Can you work these out from the model? Positions are in its coordinate system, mm. A direction names the side the tool comes from. Give positions to 0.01 mm unless a question says otherwise; leave off trailing zeros. Order: outer loops, then holes, each group sorted by start corner. A loop starts at its lowest first (then second) coordinate and runs counter-clockwise, first axis right, second up. Notation, with made-up numbers: (50, -3) - (76, -3) arc R32 cw to (76, 30) - close; hole circle Ø3 at (58, 86.5). An arc over 180 degrees is marked (long way). Answer as CSV lines item,"result".
```python
from build123d import *

# Parameters (mm, degrees)
SKETCH1_W                      = 55
SKETCH1_H                      = 39.55
SKETCH1_R                      = 7.5
BOSS_EXTRUDE1_DEPTH            = 45
SKETCH3_R                      = 4
CUT_EXTRUDE1_DEPTH             = 9.55
SKETCH4_W                      = 11
SKETCH4_H                      = 20
CUT_EXTRUDE2_DEPTH             = 65.21216785
M3_CLEARANCE_HOLE1_D           = 3.4
M3_CLEARANCE_HOLE1_DEPTH       = 32
M3_CLEARANCE_HOLE1_CSINK_D     = 3.45
M3_CLEARANCE_HOLE1_CSINK_ANGLE = 90
M3_CLEARANCE_HOLE1_TIP         = 1.021463052
SKETCH8_W                      = 9
SKETCH8_H                      = 4.627198444
CUT_EXTRUDE3_DEPTH             = 65.21216785
FILLET1_R                      = 10
FILLET2_R                      = 2
FILLET3_R                      = 6
FILLET4_R                      = 13


with BuildPart() as part:
    # Sketch1 → Boss-Extrude1 (new body)
    with BuildSketch(Plane.XY):
        with Locations((-7.5, 9.775)):
            Rectangle(SKETCH1_W, SKETCH1_H)
        with Locations((7.34, 19.55)):
            Circle(SKETCH1_R, mode=Mode.SUBTRACT)
    extrude(amount=-BOSS_EXTRUDE1_DEPTH)

    # Sketch3 → Cut-Extrude1 (cut)
    with BuildSketch(Plane.XZ.offset(10)):
        with Locations((7.34, -11.25)):
            Circle(SKETCH3_R)
        with Locations((7.34, -33.75)):
            Circle(SKETCH3_R)
    extrude(amount=-CUT_EXTRUDE1_DEPTH, mode=Mode.SUBTRACT)

    # Sketch4 → Cut-Extrude2 (cut, through all)
    with BuildSketch(Plane.XY):
        with Locations((-26.5, 0)):
            Rectangle(SKETCH4_W, SKETCH4_H)
    extrude(amount=-CUT_EXTRUDE2_DEPTH, mode=Mode.SUBTRACT)

    # M3 Clearance Hole1
    with Locations(Plane(origin=(-35, -1, -36), x_dir=(0, 0, -1), z_dir=(-1, 0, 0))):
        with Locations((0, 0), (-27, 0)):
            CounterSinkHole(M3_CLEARANCE_HOLE1_D / 2, M3_CLEARANCE_HOLE1_CSINK_D / 2, depth=M3_CLEARANCE_HOLE1_DEPTH, counter_sink_angle=M3_CLEARANCE_HOLE1_CSINK_ANGLE)
            with Locations((0, 0, -(M3_CLEARANCE_HOLE1_DEPTH + M3_CLEARANCE_HOLE1_TIP / 2))):  # 118° drill point
                Cone(0, M3_CLEARANCE_HOLE1_D / 2, M3_CLEARANCE_HOLE1_TIP, mode=Mode.SUBTRACT)

    # Sketch8 → Cut-Extrude3 (cut, through all)
    with BuildSketch(Plane.XY):
        with Locations((-26.66, 24.492052806)):
            Rectangle(SKETCH8_W, SKETCH8_H)
    extrude(amount=-CUT_EXTRUDE3_DEPTH, mode=Mode.SUBTRACT)

    # Fillet1
    # the kernel refuses this fillet: 10 mm, written as the material it takes off along each edge
    with BuildSketch(Plane(origin=(-46, -10, 0), x_dir=(0, 1, 0), z_dir=(1, 0, 0))) as fillet1_piece_1:
        with BuildLine():
            CenterArc((FILLET1_R, -FILLET1_R), FILLET1_R, 90, 90)
            Line((0, -FILLET1_R), (0, 0))
            Line((0, 0), (FILLET1_R, 0))
        make_face()
    extrude(amount=91, mode=Mode.SUBTRACT)
    with BuildSketch(Plane(origin=(-46, -10, -45), x_dir=(0, 1, 0), z_dir=(1, 0, 0))) as fillet1_piece_2:
        with BuildLine():
            CenterArc((FILLET1_R, FILLET1_R), FILLET1_R, 180, 90)
            Line((0, FILLET1_R), (0, 0))
            Line((0, 0), (FILLET1_R, 0))
        make_face()
    extrude(amount=91, mode=Mode.SUBTRACT)
    with BuildSketch(Plane(origin=(-60, -10, 0), x_dir=(0, 1, 0), z_dir=(1, 0, 0))) as fillet1_piece_3:
        with BuildLine():
            CenterArc((FILLET1_R, -FILLET1_R), FILLET1_R, 90, 90)
            Line((0, -FILLET1_R), (0, 0))
            Line((0, 0), (FILLET1_R, 0))
        make_face()
    extrude(amount=53, mode=Mode.SUBTRACT)
    with BuildSketch(Plane(origin=(-60, -10, -45), x_dir=(0, 1, 0), z_dir=(1, 0, 0))) as fillet1_piece_4:
        with BuildLine():
            CenterArc((FILLET1_R, FILLET1_R), FILLET1_R, 180, 90)
            Line((0, FILLET1_R), (0, 0))
            Line((0, 0), (FILLET1_R, 0))
        make_face()
    extrude(amount=53, mode=Mode.SUBTRACT)

    # Fillet2
    fillet2_edges = [part.edges().sort_by_distance(p)[0] for p in [
        (-26.5, 10, -45),
        (-26.5, 10, 0),
        (-26.66, 22.178453584, -45),
        (-26.66, 22.178453584, 0),
    ]]
    fillet(fillet2_edges, radius=FILLET2_R)

    # Fillet3
    fillet3_edges = [part.edges().sort_by_distance(p)[0] for p in [
        (-35, 29.55, -22.5),
    ]]
    fillet(fillet3_edges, radius=FILLET3_R)

    # Fillet4
    fillet4_edges = [part.edges().sort_by_distance(p)[0] for p in [
        (20, 29.55, -22.5),
    ]]
    fillet(fillet4_edges, radius=FILLET4_R)


solid = part.part
```
1) I need wall thicknesses on line 1 along X through (y, z) = (-3, -33.5); line 2 along Z through (x, y) = (6.5, -4); line 3 along Z through (x, y) = (4, -4.5). Which ranges of each line are inside material? Lowest first, please. Write a range as [from, to].
Answer block:
line 1,"[-35, -32], [-21, 3.35], [11.33, 20]"
line 2,"[-44.17, -37.66], [-29.84, -15.16], [-7.34, -0.83]"
line 3,"[-43.93, -35.95], [-31.55, -13.45], [-9.05, -1.07]"
2) I want a section at A-A on y = 4. Write out the boundary of the cut face in (x, z), plus the area to 3 significant figures.
Answer block:
outline,"(-35, -45) - (-32, -45) - (-32, 0) - (-35, 0) - close; (-21, -45) - (20, -45) - (20, 0) - (-21, 0) - close"
area,"1,980 mm2"
3) I want a section at B-B on x = -24. Write out the boundary of the cut face in (y, z).
Answer block:
outline,"(10, -43) arc R2 ccw to (12, -45) - (20.18, -45) arc R2 ccw to (22.18, -43) - (22.18, -2) arc R2 ccw to (20.18, 0) - (12, 0) arc R2 ccw to (10, -2) - close; (26.81, -45) - (29.55, -45) - (29.55, 0) - (26.81, 0) - close"
4) I want a section at D-D on z = -13. Write out the boundary of the cut face in (x, y).
Answer block:
outline,"(-35, -10) - (-32, -10) - (-32, 10) - (-21, 10) - (-21, -10) - (3.74, -10) - (3.74, -0.45) - (10.94, -0.45) - (10.94, -10) - (20, -10) - (20, 16.55) arc R13 ccw to (7, 29.55) - (-29, 29.55) arc R6 ccw to (-35, 23.55) - close; hole (-31.16, 22.18) - (-22.16, 22.18) - (-22.16, 26.81) - (-31.16, 26.81) - close; hole circle Ø15 at (7.34, 19.55)"
5) I'm going to push flat-ended pins straight in: P1, Ø10, axis at x = -26.5, z = -25.5, coming from the -Y side; P2, Ø2.5, axis at x = 7, z = -33, coming from the -Y side; P3, Ø13.5, axis at x = 7.34, y = 19.55, coming from the -Z side; P4, Ø7.5, axis at y = 23.5, z = -31.5, coming from the +X side. Where does each tip first touch, or does it pass through?
Answer block:
P1,"y = 10"
P2,"y = -0.45"
P3,"through"
P4,"x = 19.6"
6) Which directions (+Z, -Z, +X, -X, +Y, -Y) give clear straight access to the entire face, cutting with the end or side of a thin tool? Please do faces 4 (the cylindrical face through (9.49, -5.292, -30.377)), 5 (the flat face through (-34, -10, -22)), 6 (the flat face through (-27, 22.178, -22)).
Answer block:
face 4,"-Y"
face 5,"+Z, -Z, +X, -X, -Y"
face 6,"+Z, -Z"
7) I want a section at C-C on y = -6. Write out the boundary of the cut face in (x, z).
Answer block:
outline,"(-35, -43) - (-32, -43) - (-32, -2) - (-35, -2) - close; (-21, -43) - (20, -43) - (20, -2) - (-21, -2) - close; hole circle Ø8 at (7.34, -33.75); hole circle Ø8 at (7.34, -11.25)"
8) If we mould it in two halves opening along Y, with no side actions, what happens to faces 1 (the cylindrical face through (-11.87, -2.15, -10.25)), 2 (the flat face through (7, -0.45, -11)), 3 (the flat face through (-35, 7, -22))? For each: +Y half, -Y half, draft (parallel to the pull), parting line (faces both ways), or undercut.
Answer block:
face 1,"undercut"
face 2,"-Y half"
face 3,"draft"
